Check sheet for the modelled part. Datum: model origin and axes. Units: mm. A direction names the side the tool comes from. Round coordinates to 2 decimals unless told otherwise and drop trailing zeros. Order: outer loops, then holes, each group sorted by start corner. A loop starts at its lowest first (then second) coordinate and runs counter-clockwise, first axis right, second up.
Autodesk Inventor part; units mm, degrees
ref_plane "YZ Plane" through (0, 0, 0) normal (1, 0, 0) x (0, 1, 0)
ref_plane "XZ Plane" through (0, 0, 0) normal (0, 1, 0) x (-1, 0, 0)
ref_plane "XY Plane" through (0, 0, 0) normal (0, 0, 1) x (1, 0, 0)
sketch "Sketch1" plane through (0, 0, 0) normal (0, 1, 0) x (-1, 0, 0)
  circle A0 centre (0, 0) radius 2.75
  circle A1 centre (0, 0) radius 2
  dimension "d0" = 5.5
  dimension "d1" = 4
extrude "Extrusion1" add sketch "Sketch1" against normal blind 10 contours A1
extrude "Extrusion2" add sketch "Sketch1" along normal blind 2.8 contours A0 | A1
sketch "Sketch2" plane through (0, 2.8, 0) normal (0, 1, 0) x (1, 0, 0)
  circle A0 centre (0, 0) radius 2
  line L0 (-1.25, -0.7217) -> (-1.25, 0.7217)
  line L1 (-1.25, 0.7217) -> (0, 1.4434)
  line L2 (0, 1.4434) -> (1.25, 0.7217)
  line L3 (1.25, 0.7217) -> (1.25, -0.7217)
  line L4 (1.25, -0.7217) -> (0, -1.4434)
  line L5 (0, -1.4434) -> (-1.25, -0.7217)
  dimension "d6" = 2.5
extrude "Extrusion3" cut sketch "Sketch2" against normal blind 2 contours L0 L1 L2 L3 L4 L5
equation "\"d0\" = D_"
equation "\"d1\" = M_"
equation "\"d2\" = L_"
equation "\"d4\" = K_"
equation "\"d6\" = S_"
equation "\"d7\" = t_"
equation "\"K_\" = 2.8"
equation "\"D_\" = 5.5"
equation "\"S_\" = 2.5"
equation "\"t_\" = 2"
equation "\"M_\" = 4"
equation "\"L_\" = 10"
properties part number "M4 x 10" material "Stainless Steel"
1) Gauge pin test, flat ends, axial feed: pin 1 (2 mm diameter, centred on x = -0.5, z = -0.5, fed in from +Y); pin 2 (3 mm diameter, centred on x = 0, y = -7, fed in from +Z); pin 3 (3 mm diameter, centred on y = -2, z = -0.5, fed in from -X). Record the tip position at first contact, or that the pin passes through.
2) Sectioned sample at B-B on z = 0. Record the cut outline in (x, y).
3) Set-up check for faces 1 (the face through (0.63, 1.81, 1.08)), 2 (the face through (0.596, 1.38, 2.685)), 3 (the face through (-1, 0, -2)): record each of +Z, -Z, +X, -X, +Y, -Y from which the full face is reachable in a straight line by a thin tool's end or side.
4) Sectioned sample at C-C on x = -1.1. Record the cut outline in (y, z), and give its area (3 significant figures).
5) Sectioned sample at A-A on y = 1.5. Record the cut outline in (x, z), and give its area (3 significant figures).
6) Draft check along X on faces 4 (the face through (0, 0.8, 0)), 5 (the face through (0, -10, 0)), 6 (the face through (1.25, 2, 0)), 7 (the face through (0, -5, -2)). Enter one of: pulls with the +X half, pulls with the -X half, needs draft (parallel to the pull), parting line crosses it, or undercut.
7) Scan lines: line 1 (Y direction, x = -0.45, z = -0.8); line 2 (X direction, y = -9.25, z = -0.1); line 3 (X direction, y = 1.25, z = -1.3). Record each from-to range of solid material in increasing order.
8) Sectioned sample at D-D on y = -8.5. Record the cut outline in (x, z), and give its area (3 significant figures).
Values found:
1. pin 1: stops at y = 2.8
1. pin 2: stops at z = 2
1. pin 3: stops at x = -2
2. outline: (-2.75, 0) - (-2, 0) - (-2, -10) - (2, -10) - (2, 0) - (2.75, 0) - (2.75, 2.8) - (1.25, 2.8) - (1.25, 0.8) - (-1.25, 0.8) - (-1.25, 2.8) - (-2.75, 2.8) - close
3. face 1: +Y
3. face 2: +Y, -Y
3. face 3: -Y
4. outline: (-10, -1.67) - (0, -1.67) - (0, -2.52) - (2.8, -2.52) - (2.8, -0.81) - (0.8, -0.81) - (0.8, 0.81) - (2.8, 0.81) - (2.8, 2.52) - (0, 2.52) - (0, 1.67) - (-10, 1.67) - close
4. area: 44.3 mm2
5. outline: circle Ø5.5 at (0, 0); hole (-1.25, -0.72) - (0, -1.44) - (1.25, -0.72) - (1.25, 0.72) - (0, 1.44) - (-1.25, 0.72) - close
5. area: 18.3 mm2
6. face 4: undercut
6. face 5: needs draft
6. face 6: undercut
6. face 7: parting line crosses it
7. line 1: y = -10 to 0.8
7. line 2: x = -2 to 2
7. line 3: x = -2.42 to -0.25, 0.25 to 2.42
8. outline: circle Ø4 at (0, 0)
8. area: 12.6 mm2
